For this review, take the finished solid that the model builds, in its own axes (mm). Coordinates: 2 decimals unless noted, no trailing zeros. Order: outer loops, then holes, each group sorted by start corner. A loop starts at its lowest first (then second) coordinate and runs counter-clockwise, first axis right, second up. Notation, with made-up numbers: M -3,-36.5 L 10,-36.5 A19 cw 10,-30.5 Z; hole C -24,-39 d5. An arc over 180 degrees is marked long. Use CSV: the item, a comma, the result in double quotes.
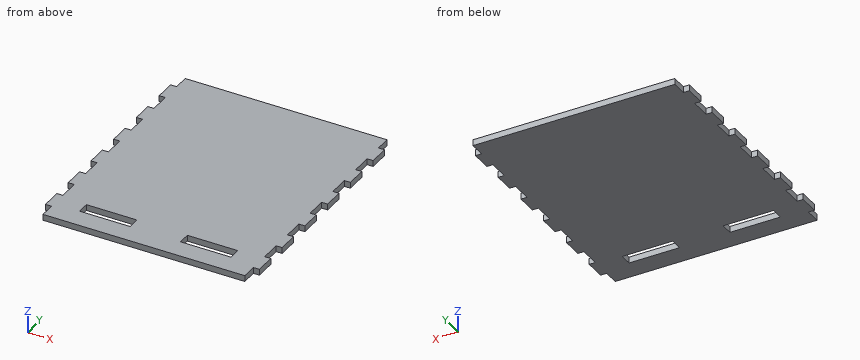
```python
from build123d import *

# Parameters (mm, degrees)
SKETCH_1_W      = 50
SKETCH_1_H      = 12
EXTRUDE_1_DEPTH = 6


with BuildPart() as part:
    # 草图1 → 凸台-拉伸1 (new body)
    with BuildSketch(Plane.XY):
        Polygon((-118.430922138, 110.033611019), (-118.430922138, 90.033611019), (-124.430922138, 90.033611019), (-124.430922138, 70.033611019), (-118.430922138, 70.033611019), (-118.430922138, 50.033611019), (-124.430922138, 50.033611019), (-124.430922138, 30.033611019), (-118.430922138, 30.033611019), (-118.430922138, 10.033611019), (-124.430922138, 10.033611019), (-124.430922138, -9.966388981), (-118.430922138, -9.966388981), (-118.430922138, -29.966388981), (-124.430922138, -29.966388981), (-124.430922138, -49.966388981), (-118.430922138, -49.966388981), (-118.430922138, -69.966388981), (-124.430922138, -69.966388981), (-124.430922138, -89.966388981), (-118.430922138, -89.966388981), (-118.430922138, -104.966388981), (81.569077862, -104.966388981), (81.569077862, -89.966388981), (87.569077862, -89.966388981), (87.569077862, -69.966388981), (81.569077862, -69.966388981), (81.569077862, -49.966388981), (87.569077862, -49.966388981), (87.569077862, -29.966388981), (81.569077862, -29.966388981), (81.569077862, -9.966388981), (87.569077862, -9.966388981), (87.569077862, 10.033611019), (81.569077862, 10.033611019), (81.569077862, 30.033611019), (87.569077862, 30.033611019), (87.569077862, 50.033611019), (81.569077862, 50.033611019), (81.569077862, 70.033611019), (87.569077862, 70.033611019), (87.569077862, 90.033611019), (81.569077862, 90.033611019), (81.569077862, 110.033611019), (87.569077862, 110.033611019), (87.569077862, 130.033611019), (81.569077862, 130.033611019), (81.569077862, 145.033611019), (-118.430922138, 145.033611019), (-118.430922138, 130.033611019), (-124.430922138, 130.033611019), (-124.430922138, 110.033611019), align=None)
        with Locations((-68.430922138, -78.966388981)):
            Rectangle(SKETCH_1_W, SKETCH_1_H, mode=Mode.SUBTRACT)
        with Locations((31.569077862, -78.966388981)):
            Rectangle(SKETCH_1_W, SKETCH_1_H, mode=Mode.SUBTRACT)
    extrude(amount=EXTRUDE_1_DEPTH)


solid = part.part
```
Item 1: Clearance check with flat-ended pins moving along their axes: pin 1 Ø1 at (y, z) = (-23, 4.5) entering from +X; pin 2 Ø3 at (x, z) = (83.5, 2.5) entering from +Y; pin 3 Ø3 at (y, z) = (-24, 2.5) entering from -X. State where each tip first meets the part, or that it passes through.
Solutions:
pin 1,"x = 81.57"
pin 2,"y = 130.03"
pin 3,"x = -118.43"
Item 2: To check wall thickness, follow line 1 along X through (y, z) = (-74, 4.6); line 2 along Y through (x, z) = (52, 4.45); line 3 along X through (y, z) = (-24, 1.65). State the ranges of each line that lie inside material, in increasing order. Write a range as [from, to].
Solutions:
line 1,"[-124.43, -93.43], [-43.43, 6.57], [56.57, 87.57]"
line 2,"[-104.97, -84.97], [-72.97, 145.03]"
line 3,"[-118.43, 81.57]"
Item 3: Add section B-B on z = 2.45. State how many separate pieces and enclosed holes the cut face has, and give its area (3 significant figures).
Solutions:
separate pieces,"1"
enclosed holes,"2"
area,"50,200 mm^2"
Item 4: Add section C-C on y = 98. State the section outline as (x, z) points, and give its area (3 significant figures).
Solutions:
outline,"M -118.43,0 L 81.57,0 L 81.57,6 L -118.43,6 Z"
area,"1,200 mm^2"
Item 5: Add section A-A on x = 51.5. State the section outline as (y, z) points, and give its area (3 significant figures).
Solutions:
outline,"M -104.97,0 L -84.97,0 L -84.97,6 L -104.97,6 Z; M -72.97,0 L 145.03,0 L 145.03,6 L -72.97,6 Z"
area,"1,430 mm^2"
